```python
from build123d import *

# Parameters (mm, degrees)
SKETCH1_W           = 42
SKETCH1_H           = 42
BOSS_EXTRUDE1_DEPTH = 23
CHAMFER1_SIZE       = 3
CUT_EXTRUDE_2_REACH = 25
SKETCH4_R           = 1.8
CUT_EXTRUDE_3_REACH = 25
SKETCH2_R           = 14


with BuildPart() as part:
    # Sketch1 → Boss-Extrude1 (new body)
    with BuildSketch(Plane.XY):
        Rectangle(SKETCH1_W, SKETCH1_H)
    extrude(amount=BOSS_EXTRUDE1_DEPTH)

    # Chamfer1
    chamfer1_edges = [part.edges().sort_by_distance(p)[0] for p in [
        (21, -21, 11.5),
        (-21, -21, 11.5),
        (-21, 21, 11.5),
        (21, 21, 11.5),
    ]]
    chamfer(chamfer1_edges, length=CHAMFER1_SIZE)

    # Sketch4 → Вырез-Вытянуть2 (cut, up to next)
    with BuildSketch(Plane.XY.offset(23), mode=Mode.PRIVATE) as cut_extrude_2_sk1:
        with Locations((-15.75, 15.75)):
            Circle(SKETCH4_R)
    cut_extrude_2_tool1 = extrude(cut_extrude_2_sk1.sketch, amount=-CUT_EXTRUDE_2_REACH, mode=Mode.PRIVATE) & part.part
    add(cut_extrude_2_tool1.solids().sort_by_distance((-15.75, 15.75, 23))[0], mode=Mode.SUBTRACT)
    # Sketch4 → Вырез-Вытянуть2 (cut, up to next)
    with BuildSketch(Plane.XY.offset(23), mode=Mode.PRIVATE) as cut_extrude_2_sk2:
        with Locations((15.75, 15.75)):
            Circle(SKETCH4_R)
    cut_extrude_2_tool2 = extrude(cut_extrude_2_sk2.sketch, amount=-CUT_EXTRUDE_2_REACH, mode=Mode.PRIVATE) & part.part
    add(cut_extrude_2_tool2.solids().sort_by_distance((15.75, 15.75, 23))[0], mode=Mode.SUBTRACT)
    # Sketch4 → Вырез-Вытянуть2 (cut, up to next)
    with BuildSketch(Plane.XY.offset(23), mode=Mode.PRIVATE) as cut_extrude_2_sk3:
        with Locations((-15.75, -15.75)):
            Circle(SKETCH4_R)
    cut_extrude_2_tool3 = extrude(cut_extrude_2_sk3.sketch, amount=-CUT_EXTRUDE_2_REACH, mode=Mode.PRIVATE) & part.part
    add(cut_extrude_2_tool3.solids().sort_by_distance((-15.75, -15.75, 23))[0], mode=Mode.SUBTRACT)
    # Sketch4 → Вырез-Вытянуть2 (cut, up to next)
    with BuildSketch(Plane.XY.offset(23), mode=Mode.PRIVATE) as cut_extrude_2_sk4:
        with Locations((15.75, -15.75)):
            Circle(SKETCH4_R)
    cut_extrude_2_tool4 = extrude(cut_extrude_2_sk4.sketch, amount=-CUT_EXTRUDE_2_REACH, mode=Mode.PRIVATE) & part.part
    add(cut_extrude_2_tool4.solids().sort_by_distance((15.75, -15.75, 23))[0], mode=Mode.SUBTRACT)

    # Sketch2 → Вырез-Вытянуть3 (cut, up to next)
    with BuildSketch(Plane.XY.offset(23), mode=Mode.PRIVATE) as cut_extrude_3_sk1:
        Circle(SKETCH2_R)
    cut_extrude_3_tool1 = extrude(cut_extrude_3_sk1.sketch, amount=-CUT_EXTRUDE_3_REACH, mode=Mode.PRIVATE) & part.part
    add(cut_extrude_3_tool1.solids().sort_by_distance((0, 0, 23))[0], mode=Mode.SUBTRACT)


solid = part.part
```
Geometry check sheet. Reference: the model listing, model coordinates, mm. Coordinates: 2 decimals unless noted, no trailing zeros. Order: outer loops, then holes, each group sorted by start corner. A loop starts at its lowest first (then second) coordinate and runs counter-clockwise, first axis right, second up. Notation, with made-up numbers: M 89,18.5 L 100,18.5 A21 ccw 100,56.5 Z; hole C -17,36 d6. An arc over 180 degrees is marked long. Answer as a JSON object with one key per item and string values.
Q1. Scan lines: line 1 (Y direction, x = -15.75, z = 14.75); line 2 (Y direction, x = -11.5, z = 4.25); line 3 (X direction, y = -16, z = 15). Record each from-to range of solid material in increasing order.
Results are:
{"line 1": "y = -21 to -17.55, -13.95 to 13.95, 17.55 to 21", "line 2": "y = -21 to -7.98, 7.98 to 21", "line 3": "x = -21 to -17.53, -13.97 to 13.97, 17.53 to 21"}
Q2. Release check for a two-part mould opening along Y. For faces 1 (the flat face through (20, -19, 11)), 2 (the flat face through (-21, 0, 11)), 3 (the cylindrical face through (15.516, -13.965, 11.661)) record: released by +Y, released by -Y, zero draft, split by the parting line, or undercut.
Results are:
{"face 1": "released by -Y", "face 2": "zero draft", "face 3": "undercut"}
Q3. Cross-section at D-D on z = 1.5. Record the cut outline in (x, y).
Results are:
{"outline": "M -21,-18 L -18,-21 L 18,-21 L 21,-18 L 21,18 L 18,21 L -18,21 L -21,18 Z; hole C -15.75,-15.75 d3.6; hole C -15.75,15.75 d3.6; hole C 0,0 d28; hole C 15.75,-15.75 d3.6; hole C 15.75,15.75 d3.6"}
Q4. Cross-section at B-B on x = 15.75. Record the cut outline in (y, z).
Results are:
{"outline": "M -21,0 L -17.55,0 L -17.55,23 L -21,23 Z; M -13.95,0 L 13.95,0 L 13.95,23 L -13.95,23 Z; M 17.55,0 L 21,0 L 21,23 L 17.55,23 Z"}
Q5. Cross-section at A-A on x = 0. Record the cut outline in (y, z).
Results are:
{"outline": "M -21,0 L -14,0 L -14,23 L -21,23 Z; M 14,0 L 21,0 L 21,23 L 14,23 Z"}
